Autodesk Inventor part; units mm, degrees
ref_plane "YZ Plane" through (0, 0, 0) normal (1, 0, 0) x (0, 1, 0)
ref_plane "XZ Plane" through (0, 0, 0) normal (0, 1, 0) x (-1, 0, 0)
ref_plane "XY Plane" through (0, 0, 0) normal (0, 0, 1) x (1, 0, 0)
sketch "Sketch1" plane through (0, 0, 0) normal (0, 1, 0) x (-1, 0, 0)
  line L0 (36, 23) -> (0, 23)
  line L1 (0, 23) -> (0, 0)
  line L2 (0, 0) -> (36, 0)
  line L3 (36, 0) -> (36, 23)
  dimension "d0" = 36
  dimension "d1" = 23
extrude "Extrusion1" add sketch "Sketch1" along normal blind 4.4
sketch "Sketch2" plane through (0, 4.4, 0) normal (0, 1, 0) x (1, 0, 0)
  line L0 (-36, -23) -> (0, -23)
  line L1 (-15.4, -17) -> (-7.4, -17)
  line L2 (-7.4, -17) -> (-7.4, -23)
  line L3 (-7.4, -23) -> (-15.4, -23)
  line L4 (-15.4, -23) -> (-15.4, -17)
  line L5 (0, -23) -> (0, 0)
  dimension "d4" = 8
  dimension "d5" = 6
  dimension "d6" = 7.4
extrude "Extrusion2" add sketch "Sketch2" along normal blind 3.1
properties part number "Power Booster" material "ABS Plastic"
Input: part model. Units: mm. Frame: model coordinates. A direction names the side the tool comes from. Give positions to 0.01 mm unless a question says otherwise; leave off trailing zeros. Order: outer loops, then holes, each group sorted by start corner. A loop starts at its lowest first (then second) coordinate and runs counter-clockwise, first axis right, second up. Notation, with made-up numbers: M 83.25,73 L 93.25,73 A24 cw 93.25,93 Z; hole C -34.75,26.25 d8. An arc over 180 degrees is marked long. One line per question, with ' | ' between items. Start each with the question number.
1. Access query for faces 1 (the face through (-11, 6, 17)), 2 (the face through (-15.4, 6, 20)), 3 (the face through (-18, 3, 23)), 4 (the face through (-18, 0, 12)), 5 (the face through (-7.4, 6, 20)). Directions: +Z, -Z, +X, -X, +Y, -Y. A direction counts if a zero-diameter tool reaches every point of the face in a straight line with its end or side. Return the directions, or none.
2. Section query D-D (z = 9.5). Return the cut outline in (x, y), and give its area (3 significant figures).
3. Section query C-C (y = 5.25). Return the cut outline in (x, z).
4. Material intervals for probe 1 along Y at (x, z) = (-2.5, 5.5); probe 2 along X at (y, z) = (4.75, 19.75); probe 3 along Z at (x, y) = (-13.5, 5), sorted ascending. Write a range as [from, to].
5. First-contact query: pin 1 Ø7 at (x, z) = (-15, 6.5) entering from +Y; pin 2 Ø0.9 at (y, z) = (6.5, 19) entering from -X; pin 3 Ø2.5 at (x, y) = (-11.5, 5.5) entering from -Z; pin 4 Ø0.9 at (y, z) = (6.5, 19) entering from +X. Flat tips, straight axial feed; report the tip coordinate or a pass-through.
6. Section query A-A (z = 19). Return the cut outline in (x, y), and give its area (3 significant figures).
7. Section query B-B (x = -10). Return the cut outline in (y, z).
Here are the results:
1) face 1: -Z, +X, -X, +Y | face 2: +Z, -Z, -X, +Y | face 3: +Z, +X, -X, +Y, -Y | face 4: +Z, -Z, +X, -X, -Y | face 5: +Z, -Z, +X, +Y
2) outline: M -36,0 L 0,0 L 0,4.4 L -36,4.4 Z | area: 158 mm²
3) outline: M -15.4,17 L -7.4,17 L -7.4,23 L -15.4,23 Z
4) probe 1: [0, 4.4] | probe 2: [-15.4, -7.4] | probe 3: [17, 23]
5) pin 1: y = 4.4 | pin 2: x = -15.4 | pin 3: z = 0 | pin 4: x = -7.4
6) outline: M -36,0 L 0,0 L 0,4.4 L -7.4,4.4 L -7.4,7.5 L -15.4,7.5 L -15.4,4.4 L -36,4.4 Z | area: 183 mm²
7) outline: M 0,0 L 4.4,0 L 4.4,17 L 7.5,17 L 7.5,23 L 0,23 Z
